```python
from build123d import *

# Parameters (mm, degrees)
BASE_FLANGE1_DEPTH          = 1.5
SM_EDGE_FLANGE_1_DEPTH      = 45
SM_EDGE_FLANGE_1_BEND_DEPTH = 45
SKETCH12_R                  = 3
CUT_EXTRUDE1_DEPTH          = 10
FILLET1_R                   = 10
SKETCH13_R                  = 3
CUT_EXTRUDE2_DEPTH          = 10
SKETCH14_R                  = 2
CUT_EXTRUDE3_DEPTH          = 10


# Sheet-metal steps are written as plain solids
with BuildPart() as part:
    # Sketch1 → Base-Flange1 (new body)
    with BuildSketch(Plane.XY):
        with BuildLine():
            Line((15, 0), (134, 0))
            ThreePointArc((134, 0), (144.606601718, 4.393398282), (149, 15))
            Line((149, 15), (149, 70))
            ThreePointArc((149, 70), (144.606601718, 80.606601718), (134, 85))
            Line((134, 85), (15, 85))
            ThreePointArc((15, 85), (4.393398282, 80.606601718), (0, 70))
            Line((0, 70), (0, 15))
            ThreePointArc((0, 15), (4.393398282, 4.393398282), (15, 0))
        make_face()
        with BuildLine():
            Line((111.5, 15), (37.5, 15))
            ThreePointArc((37.5, 15), (28.307611845, 18.807611845), (24.5, 28))
            Line((24.5, 28), (24.5, 57))
            ThreePointArc((24.5, 57), (28.307611845, 66.192388155), (37.5, 70))
            Line((37.5, 70), (111.5, 70))
            ThreePointArc((111.5, 70), (120.692388155, 66.192388155), (124.5, 57))
            Line((124.5, 57), (124.5, 28))
            ThreePointArc((124.5, 28), (120.692388155, 18.807611845), (111.5, 15))
        make_face(mode=Mode.SUBTRACT)
    extrude(amount=-BASE_FLANGE1_DEPTH)

    # Ребро-кромка1 section (across the edge) → Ребро-кромка1 (add)
    with BuildSketch(Plane(origin=(-0.495706006, 20, -1.5), x_dir=(0.49999999999999495, 0, -0.8660254037844416), z_dir=(0, 1, 0))):
        with BuildLine():
            Line((-1.5, 0.495706006), (-1.5, 39.598076211))
            Line((-1.5, 39.598076211), (0, 39.598076211))
            Line((0, 39.598076211), (0, 0.495706006))
            ThreePointArc((0, 0.495706006), (0.063037221, 0.016890773), (0.247853003, -0.429293994))
            Line((0.247853003, -0.429293994), (-1.051185103, -1.179293994))
            ThreePointArc((-1.051185103, -1.179293994), (-1.385851518, -0.371337795), (-1.5, 0.495706006))
        make_face()
    extrude(amount=SM_EDGE_FLANGE_1_DEPTH)

    # Ребро-кромка1 section 2 (across the edge) → Ребро-кромка1 bend (add)
    with BuildSketch(Plane(origin=(149.495706006, 65, -1.5), x_dir=(-0.49999999999999495, 0, -0.8660254037844416), z_dir=(0, -1, 0))):
        with BuildLine():
            Line((-1.5, 0.495706006), (-1.5, 39.598076211))
            Line((-1.5, 39.598076211), (0, 39.598076211))
            Line((0, 39.598076211), (0, 0.495706006))
            ThreePointArc((0, 0.495706006), (0.063037221, 0.016890773), (0.247853003, -0.429293994))
            Line((0.247853003, -0.429293994), (-1.051185103, -1.179293994))
            ThreePointArc((-1.051185103, -1.179293994), (-1.385851518, -0.371337795), (-1.5, 0.495706006))
        make_face()
    extrude(amount=SM_EDGE_FLANGE_1_BEND_DEPTH)

    # Sketch12 → Cut-Extrude1 (cut)
    with BuildSketch(Plane(origin=(37.474407449, 0, 64.907577685), x_dir=(0.8660254037844416, 0, -0.49999999999999517), z_dir=(0.49999999999999517, 0, 0.8660254037844416))):
        with Locations((161.815155369, 30)):
            Circle(SKETCH12_R)
        with Locations((161.815155369, 55)):
            Circle(SKETCH12_R)
    extrude(amount=-CUT_EXTRUDE1_DEPTH, mode=Mode.SUBTRACT)

    # Fillet1
    fillet1_edges = [part.edges().sort_by_distance(p)[0] for p in [
        (-35.163645946, 20, -20.649519053),
        (-35.163645946, 65, -20.649519053),
        (184.163645946, 65, -20.649519053),
        (184.163645946, 20, -20.649519053),
    ]]
    fillet(fillet1_edges, radius=FILLET1_R)

    # Sketch13 → Cut-Extrude2 (cut)
    with BuildSketch(Plane(origin=(-0.224407449, 0, 0.388685103), x_dir=(0.8660254037844416, 0, 0.49999999999999517), z_dir=(-0.49999999999999517, 0, 0.8660254037844416))):
        with Locations((-32.777370205, 30)):
            Circle(SKETCH13_R)
        with Locations((-32.777370205, 55)):
            Circle(SKETCH13_R)
    extrude(amount=-CUT_EXTRUDE2_DEPTH, mode=Mode.SUBTRACT)

    # Sketch14 → Cut-Extrude3 (cut)
    with BuildSketch(Plane(origin=(0, 0, -1.5), x_dir=(-1, 0, 0), z_dir=(0, 0, -1))):
        with Locations((-138.5, 42.5)):
            Circle(SKETCH14_R)
        with Locations((-10.5, 42.5)):
            Circle(SKETCH14_R)
    extrude(amount=-CUT_EXTRUDE3_DEPTH, mode=Mode.SUBTRACT)


solid = part.part
```
Source: CAD feature listing. Evaluate the final solid. Frame: model axes, mm. A direction names the side the tool comes from. Round coordinates to 2 decimals unless told otherwise and drop trailing zeros. Order: outer loops, then holes, each group sorted by start corner. A loop starts at its lowest first (then second) coordinate and runs counter-clockwise, first axis right, second up. Notation, with made-up numbers: (-19, -6) -> (-12, -6) arc R18 ccw to (-12, 4) -> close; hole circle Ø2 at (-10, -28). An arc over 180 degrees is marked (long way). Use CSV: the item, a comma, the result in double quotes.
(1) Section C-C on z = -7.5. Return the cut outline in (x, y).
Report:
outline,"(-13.89, 20) -> (-10.89, 20) -> (-10.89, 65) -> (-13.89, 65) -> close; (159.89, 20) -> (162.89, 20) -> (162.89, 65) -> (159.89, 65) -> close"
(2) Section B-B on x = 46.5. Return the cut outline in (y, z), and give its area (3 significant figures).
Report:
outline,"(0, -1.5) -> (15, -1.5) -> (15, 0) -> (0, 0) -> close; (70, -1.5) -> (85, -1.5) -> (85, 0) -> (70, 0) -> close"
area,"45.0 mm^2"
(3) Pull-direction query (Y, two-part tool) for faces 3 (the face through (73, 71, -1.5)), 4 (the face through (28.207, 66.091, -0.74)), 5 (the face through (-32.55, 62.15, -19.16)), 6 (the face through (-32.55, 22.85, -19.16)); classes: +Y half, -Y half, draft (parallel to the pull), parting line (faces both ways), or undercut.
Report:
face 3,"draft"
face 4,"undercut"
face 5,"+Y half"
face 6,"-Y half"
(4) Access query for faces 1 (the face through (120.793, 18.909, -0.74)), 2 (the face through (144.49, 4.28, -0.74)). Directions: +Z, -Z, +X, -X, +Y, -Y. A direction counts if a zero-diameter tool reaches every point of the face in a straight line with its end or side. Return the directions, or none.
Report:
face 1,"+Z, -Z"
face 2,"+Z, -Z, +X, -Y"
(5) Section A-A on y = 48. Return the cut outline in (x, z) (3 decimals).
Report:
outline,"(-35.539, -20) -> (-34.789, -21.299) -> (-0.925, -1.748) arc R1.85 cw to (0, -1.5) -> (24.5, -1.5) -> (24.5, 0) -> (0, 0) arc R3.35 ccw to (-1.675, -0.449) -> close; (124.5, -1.5) -> (149, -1.5) arc R1.85 cw to (149.925, -1.748) -> (183.789, -21.299) -> (184.539, -20) -> (150.675, -0.449) arc R3.35 ccw to (149, 0) -> (124.5, 0) -> close"
(6) Section D-D on x = 17. Return the cut outline in (y, z), and give its area (4 significant figures).
Report:
outline,"(0, -1.5) -> (85, -1.5) -> (85, 0) -> (0, 0) -> close"
area,"127.5 mm^2"
(7) First-contact query: pin 1 Ø3.5 at (x, y) = (10.5, 42.5) entering from -Z; pin 2 Ø0.5 at (y, z) = (18.5, -0.5) entering from +X; pin 3 Ø1.5 at (x, z) = (159.5, -7.5) entering from +Y; pin 4 Ø0.8 at (y, z) = (42, -0.5) entering from +X. Flat tips, straight axial feed; report the tip coordinate or a pass-through.
Report:
pin 1,"through"
pin 2,"x = 149"
pin 3,"y = 65"
pin 4,"x = 151.46"
(8) Ray query, L1, parallel to Z at x = 84.5, y = 8; L2, parallel to X at y = 43, z = -11.25; L3, parallel to X at y = 29, z = -14. Return the intervals inside material, ascending.
Report:
L1,"-1.5 to 0"
L2,"-20.38 to -17.38, 166.38 to 169.38"
L3,"-25.15 to -22.15, 171.15 to 174.15"
